The figure shows three views and two pictorial views of one solid part (mm, origin at its lowest corner). Answer the questions. A direction names the side the tool comes from. Give positions to 0.01 mm unless a question says otherwise; leave off trailing zeros. Order: outer loops, then holes, each group sorted by start corner. A loop starts at its lowest first (then second) coordinate and runs counter-clockwise, first axis right, second up. Notation, with made-up numbers: M -13,82.25 L 13,82.25 A14 ccw 13,106.25 Z; hole C -8.5,20 d2. An arc over 180 degrees is marked long. One line per item, written item: value. Start each with the question number.
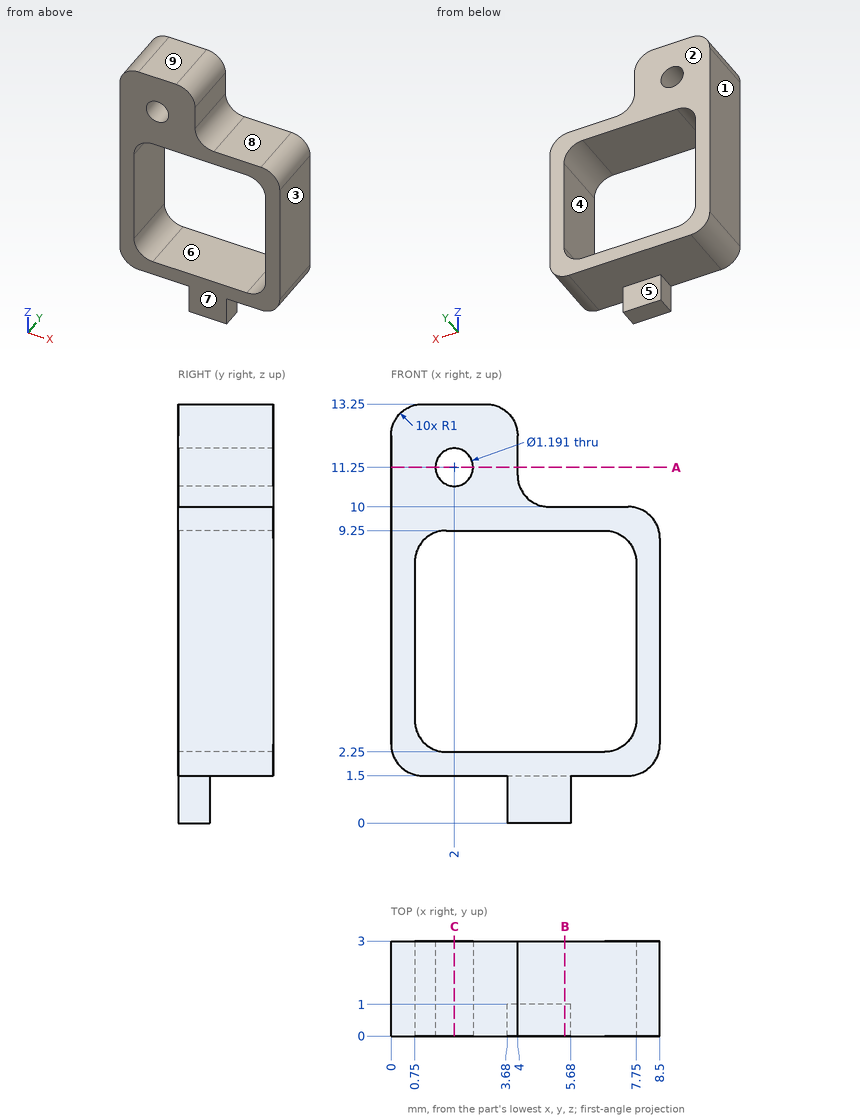
Q1. Each of these flat-tipped pins is pushed along its axis until it touches: pin 1 (0.5 mm diameter, centred on y = 0.5, z = 1, fed in from +X); pin 2 (1 mm diameter, centred on x = 3.5, z = 3, fed in from +Y); pin 3 (0.9 mm diameter, centred on x = 3, y = 1, fed in from -Z); pin 4 (0.8 mm diameter, centred on y = 0.5, z = 1, fed in from -X). Where does it stop, or does it pass through?
Q2. Find section B-B, the plane x = 5.5. Give the vertices of the cut face in (y, z).
Q3. Consider probe 1 along X at (y, z) = (2.5, 7.5); probe 2 along X at (y, z) = (1.8, 11.25) (1 decimal); probe 3 along Z at (x, y) = (2.25, 1.2). Determine where each line is inside the solid, lowest interval first.
Q4. Find section C-C, the plane x = 2. State how many separate pieces and enclosed holes the cut face has, then the cut area to 3 significant figures.
Q5. A tool of negligible diameter and unlimited length cuts with its end or side. For the marked faces 5, 6, 7, 8 and 9, from which of +Z, -Z, +X, -X, +Y, -Y can it reach the whole face along a straight path? Write none if from no direction.
Q6. Determine the mould class of the marked faces 1, 2, 3 and 4 for opening direction X: released by +X, released by -X, zero draft, split by the parting line, or undercut.
Q7. Find section A-A, the plane z = 11.25. Give the vertices of the cut face in (x, y) (1 decimal).
Evaluation:
1. pin 1: x = 5.68
1. pin 2: through
1. pin 3: z = 1.5
1. pin 4: x = 3.68
2. outline: M 0,0 L 1,0 L 1,1.5 L 3,1.5 L 3,2.25 L 0,2.25 Z; M 0,9.25 L 3,9.25 L 3,10 L 0,10 Z
3. probe 1: 0 to 0.75, 7.75 to 8.5
3. probe 2: 0 to 1.4, 2.6 to 4
3. probe 3: 1.5 to 2.25, 9.25 to 10.71, 11.79 to 13.25
4. separate pieces: 3
4. enclosed holes: 0
4. area: 10.7 mm2
5. face 5: -Z, +X, -X, +Y
5. face 6: +Y, -Y
5. face 7: +Z, -Z, +X, -X, -Y
5. face 8: +Z, +X, +Y, -Y
5. face 9: +Z, +X, -X, +Y, -Y
6. face 1: released by -X
6. face 2: zero draft
6. face 3: released by +X
6. face 4: undercut
7. outline: M 0,0 L 1.4,0 L 1.4,3 L 0,3 Z; M 2.6,0 L 4,0 L 4,3 L 2.6,3 Z
